Design review of the part built by this model. Coordinates are the model's own, in mm. Face numbers are marked on the shaded views. Give positions to 0.01 mm unless a question says otherwise; leave off trailing zeros. Loops run counter-clockwise (first coordinate to the right, second up) from the corner with the lowest first, then second, coordinate; pieces in that order, holes last. Notation, with made-up numbers: (78.5, -35.75) -> (117.5, -35.75) arc R22 ccw to (117.5, -1.75) -> close; hole circle Ø1 at (6, 62.25). An arc over 180 degrees is marked (long way). Use a Markdown table: item, result. Add a question column.
1. Draft analysis for pull direction X (two halves, no side actions). For the marked faces 1, 2 and 3, state which applies: pulls with the +X half, pulls with the -X half, needs draft (parallel to the pull), parting line crosses it, or undercut.
2. To check wall thickness, follow line 1 (X direction, y = 12.25, z = -6.5); line 2 (X direction, y = 7, z = -1.75); line 3 (X direction, y = 4.5, z = -3.5). State the ranges of each line that lie inside material, in increasing order.
3. Add section B-B (y = 3.25). State the section outline as (x, z) points (1 decimal).
4. Add section A-A (x = 0). State the section outline as (y, z) points (1 decimal).
5. For pin 1 Ø1 at (x, y) = (-1.5, 10) entering from -Z; pin 2 Ø3 at (y, z) = (7.5, -7.5) entering from +X, all flat-tipped, find the tip position at first contact; note any pin that passes through.
```python
from build123d import *

# Parameters (mm, degrees)
BOSS_EXTRUDE1_DEPTH = 12.7
CHAMFER1_SIZE       = 1.016
CHAMFER2_SIZE       = 0.635
FILLET1_R           = 0.381


with BuildPart() as part:
    # Sketch1 → Boss-Extrude1 (new body)
    with BuildSketch(Plane(origin=(0, 0, 0), x_dir=(1, 0, 0), z_dir=(0, 1, 0))):
        with BuildLine():
            ThreePointArc((-5.612660076, 5.612660076), (3.037549744, 7.333293789), (7.9375, 0))
            Line((7.9375, 0), (11.43, 0))
            ThreePointArc((11.43, 0), (4.374071632, 10.559943057), (-8.082230509, 8.082230509))
            Line((-8.082230509, 8.082230509), (-5.612660076, 5.612660076))
        make_face()
    extrude(amount=BOSS_EXTRUDE1_DEPTH)

    # Chamfer1
    chamfer1_edges = [part.edges().sort_by_distance(p)[0] for p in [
        (-6.847445292, 12.7, -6.847445292),
        (9.68375, 12.7, 0),
        (-6.847445292, 0, -6.847445292),
        (4.374071632, 0, -10.559943057),
        (9.68375, 0, 0),
        (4.374071632, 12.7, -10.559943057),
    ]]
    chamfer(chamfer1_edges, length=CHAMFER1_SIZE)

    # Chamfer2
    chamfer2_edges = [part.edges().sort_by_distance(p)[0] for p in [
        (3.037549744, 0, -7.333293789),
        (3.037549744, 12.7, -7.333293789),
    ]]
    chamfer(chamfer2_edges, length=CHAMFER2_SIZE)

    # Fillet1
    fillet1_edges = [part.edges().sort_by_distance(p)[0] for p in [
        (7.9375, 6.35, 0),
        (11.43, 6.35, 0),
        (-8.082230509, 6.35, -8.082230509),
        (-5.612660076, 6.35, -5.612660076),
    ]]
    fillet(fillet1_edges, radius=FILLET1_R)


solid = part.part
```
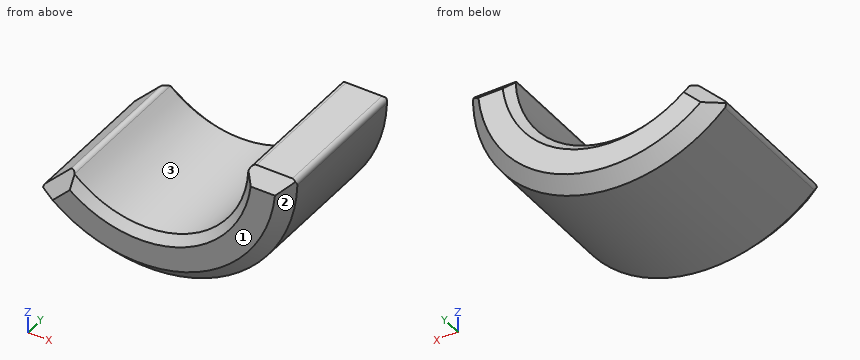
Taken from the geometry:
| question | item | result |
|---|---|---|
| 1 | face 1 | needs draft |
| 1 | face 2 | parting line crosses it |
| 1 | face 3 | undercut |
| 2 | line 1 | x = -5.7 to -4.87, 4.87 to 8.7 |
| 2 | line 2 | x = 7.74 to 11.3 |
| 2 | line 3 | x = 7.12 to 10.88 |
| 3 | outline | (-7.8, -8.4) arc R11.4 ccw to (11.4, -0.4) arc R0.4 ccw to (11, 0) -> (8.3, 0) arc R0.4 ccw to (7.9, -0.4) arc R7.9 cw to (-5.3, -5.9) arc R0.4 ccw to (-5.9, -5.9) -> (-7.8, -7.8) arc R0.4 ccw to start |
| 4 | outline | (0, -10.4) -> (1, -11.4) -> (11.7, -11.4) -> (12.7, -10.4) -> (12.7, -8.6) -> (12.1, -7.9) -> (0.6, -7.9) -> (0, -8.6) -> close |
| 5 | pin 1 | stops at z = -11.39 |
| 5 | pin 2 | stops at x = 9.73 |
